```python
from build123d import *

# Parameters (mm, degrees)
SKETCH1_W           = 85.725
SKETCH1_H           = 34.925
BOSS_EXTRUDE1_DEPTH = 3.175
SKETCH2_W           = 13.97
SKETCH2_H           = 13.97
SKETCH2_W_2         = 11.54
SKETCH2_H_2         = 12.524
CUT_EXTRUDE1_DEPTH  = 47.391954448
FILLET1_R           = 0.508
CUT_EXTRUDE2_DEPTH  = 47.391954448


with BuildPart() as part:
    # Sketch1 → Boss-Extrude1 (new body)
    with BuildSketch(Plane(origin=(0, 0, 0), x_dir=(1, 0, 0), z_dir=(0, 1, 0))):
        Rectangle(SKETCH1_W, SKETCH1_H)
    extrude(amount=BOSS_EXTRUDE1_DEPTH)

    # Sketch2 → Cut-Extrude1 (cut, through all)
    with BuildSketch(Plane(origin=(0, 0, 0), x_dir=(-1, 0, 0), z_dir=(0, -1, 0))):
        with Locations((0.8075, -1.0435)):
            Rectangle(SKETCH2_W, SKETCH2_H)
        with Locations((-29.5375, -0.3555)):
            Rectangle(SKETCH2_W_2, SKETCH2_H_2)
    extrude(amount=-CUT_EXTRUDE1_DEPTH, mode=Mode.SUBTRACT)

    # Fillet1
    fillet1_edges = [part.edges().sort_by_distance(p)[0] for p in [
        (6.1775, 1.5875, 8.0285),
        (6.1775, 1.5875, -5.9415),
        (-7.7925, 1.5875, -5.9415),
        (-7.7925, 1.5875, 8.0285),
        (23.7675, 1.5875, -5.9065),
        (23.7675, 1.5875, 6.6175),
        (35.3075, 1.5875, 6.6175),
        (35.3075, 1.5875, -5.9065),
    ]]
    fillet(fillet1_edges, radius=FILLET1_R)

    # Sketch3 → Cut-Extrude2 (cut, through all)
    with BuildSketch(Plane.XZ):
        Polygon((-26.8732, 17.4625), (-23.9268, 17.4625), (-23.9268, 13.462), (-22.987, 13.462), (-22.987, 11.811), (-23.9268, 11.811), (-23.9268, 7.8105), (-26.8732, 7.8105), (-26.8732, 11.811), (-27.813, 11.811), (-27.813, 13.462), (-26.8732, 13.462), align=None)
        Polygon((26.8732, 11.811), (26.8732, 7.8105), (23.9268, 7.8105), (23.9268, 11.811), (22.987, 11.811), (22.987, 13.462), (23.9268, 13.462), (23.9268, 17.4625), (26.8732, 17.4625), (26.8732, 13.462), (27.813, 13.462), (27.813, 11.811), align=None)
        Polygon((26.8732, -17.4625), (23.9268, -17.4625), (23.9268, -13.462), (22.987, -13.462), (22.987, -11.811), (23.9268, -11.811), (23.9268, -7.8105), (26.8732, -7.8105), (26.8732, -11.811), (27.813, -11.811), (27.813, -13.462), (26.8732, -13.462), align=None)
        Polygon((-26.8732, -11.811), (-26.8732, -7.8105), (-23.9268, -7.8105), (-23.9268, -11.811), (-22.987, -11.811), (-22.987, -13.462), (-23.9268, -13.462), (-23.9268, -17.4625), (-26.8732, -17.4625), (-26.8732, -13.462), (-27.813, -13.462), (-27.813, -11.811), align=None)
    extrude(amount=-CUT_EXTRUDE2_DEPTH, mode=Mode.SUBTRACT)


solid = part.part
```
CAD build for the part. Positions are in the model's coordinates, mm. A direction names the side the tool comes from. Give positions to 0.01 mm unless a question says otherwise; leave off trailing zeros. Order: outer loops, then holes, each group sorted by start corner. A loop starts at its lowest first (then second) coordinate and runs counter-clockwise, first axis right, second up.
(1) Saw through at C-C, the plane z = -9. Give the cut face in (x, y) (1 decimal).
(2) Saw through at B-B, the plane x = 2.5. Give the cut face in (y, z) (1 decimal), then the cut area to 3 significant figures.
(3) Mould opens along Z. For faces 1 (the flat face through (-7.792, 2, 1)), 2 (the flat face through (-25, 2, -7.81)), 3 (the flat face through (-23.927, 2, 10)) say: released by +Z, released by -Z, zero draft, split by the parting line, or undercut.
(4) Drill centre lines: L1, parallel to X at y = 0.35, z = 14.5; L2, parallel to Z at x = 27, y = 0.3; L3, parallel to Z at x = -23.5, y = 2. Where is each one in solid material? Low to high.
(5) Saw through at A-A, the plane z = 0. Give the cut face in (x, y) (1 decimal).
(6) Saw through at D-D, the plane x = 29.5. Give the cut face in (y, z) (1 decimal), then the cut area to 3 significant figures.
(7) Tool access for faces 4 (the flat face through (-35, 2, -17.462)), 5 (the flat face through (-23.927, 2, 15)), 6 (the flat face through (35, 2, 17.462)), 7 (the flat face through (27.813, 2, 13)), 8 (the flat face through (26.873, 2, -15)): list every direction of +Z, -Z, +X, -X, +Y, -Y with a clear straight run to the whole face (end or side of a thin tool).
Results found:
1. outline: (-42.9, 0) - (-26.9, 0) - (-26.9, 3.2) - (-42.9, 3.2) - close; (-23.9, 0) - (23.9, 0) - (23.9, 3.2) - (-23.9, 3.2) - close; (26.9, 0) - (42.9, 0) - (42.9, 3.2) - (26.9, 3.2) - close
2. outline: (0, -17.5) - (3.2, -17.5) - (3.2, -5.9) - (0, -5.9) - close; (0, 8) - (3.2, 8) - (3.2, 17.5) - (0, 17.5) - close
2. area: 66.5 mm2
3. face 1: undercut
3. face 2: released by -Z
3. face 3: zero draft
4. L1: x = -42.86 to -26.87, -23.93 to 23.93, 26.87 to 42.86
4. L2: z = -17.46 to -13.46, -11.81 to -5.91, 6.62 to 11.81, 13.46 to 17.46
4. L3: z = -17.46 to -13.46, -11.81 to 11.81, 13.46 to 17.46
5. outline: (-42.9, 0) - (-7.8, 0) - (-7.8, 3.2) - (-42.9, 3.2) - close; (6.2, 0) - (23.8, 0) - (23.8, 3.2) - (6.2, 3.2) - close; (35.3, 0) - (42.9, 0) - (42.9, 3.2) - (35.3, 3.2) - close
6. outline: (0, -17.5) - (3.2, -17.5) - (3.2, -5.9) - (0, -5.9) - close; (0, 6.6) - (3.2, 6.6) - (3.2, 17.5) - (0, 17.5) - close
6. area: 71.1 mm2
7. face 4: -Z, +X, -X, +Y, -Y
7. face 5: +Z, +Y, -Y
7. face 6: +Z, +X, -X, +Y, -Y
7. face 7: +Y, -Y
7. face 8: -Z, +Y, -Y
